```python
from build123d import *

# Parameters (mm, degrees)
PAD001_DEPTH     = 30
SKETCH003_W      = 15
SKETCH003_H      = 15
POCKET001_DEPTH  = 11.301
SKETCH004_R      = 2.5
PAD002_DEPTH     = 30
HOLE_D           = 4
HOLE_CSINK_D     = 8
HOLE_CSINK_ANGLE = 90
SKETCH006_R      = 2.65
POCKET002_DEPTH  = 30.001
FILLET001_R      = 1


with BuildPart() as part:
    # Sketch002 → Pad001 (new body)
    with BuildSketch(Plane.XY):
        with BuildLine():
            Line((120, 0), (138, 0))
            Line((138, 0), (138, 4))
            Line((138, 4), (125.403702, 4))
            ThreePointArc((125.403702, 4), (116.638453, 10.1912), (120, 0))
        make_face()
    extrude(amount=PAD001_DEPTH)

    # Sketch003 (on Face1 of Pad001) → Pocket001 (cut, through all)
    with BuildSketch(Plane.XZ):
        with Locations((118.3, 29.625)):
            Rectangle(SKETCH003_W, SKETCH003_H)
        with Locations((118.3, 0.375)):
            Rectangle(SKETCH003_W, SKETCH003_H)
    extrude(amount=-POCKET001_DEPTH, mode=Mode.SUBTRACT)

    # Sketch004 → Pad002 (join)
    with BuildSketch(Plane.XY):
        with Locations((120, 5.65)):
            Circle(SKETCH004_R)
    extrude(amount=PAD002_DEPTH)

    # Hole (through all)
    with Locations(Plane(origin=(0, 4, 0), x_dir=(-1, 0, 0), z_dir=(0, 1, 0))):
        with Locations((-131.9, 22.5), (-131.9, 7.5)):
            CounterSinkHole(HOLE_D / 2, HOLE_CSINK_D / 2, counter_sink_angle=HOLE_CSINK_ANGLE)

    # Sketch006 → Pocket002 (cut, through all)
    with BuildSketch(Plane.XY.offset(30)):
        with Locations((120, 5.65)):
            Circle(SKETCH006_R)
    extrude(amount=-POCKET002_DEPTH, mode=Mode.SUBTRACT)

    # Fillet001
    fillet001_edges = [part.edges().sort_by_distance(p)[0] for p in [
        (138, 4, 15),
        (131.9, 4, 0),
        (125.8, 4, 3.9375),
        (125.8, 4, 26.0625),
        (131.9, 4, 30),
    ]]
    fillet(fillet001_edges, radius=FILLET001_R)


solid = part.part
```
Here's how the part is built. I have some questions about the finished solid (model axes, mm). A direction names the side the tool comes from. Coordinates: 2 decimals unless noted, no trailing zeros. Order: outer loops, then holes, each group sorted by start corner. A loop starts at its lowest first (then second) coordinate and runs counter-clockwise, first axis right, second up. Notation, with made-up numbers: (21, 68) - (70, 68) arc R26 cw to (70, 83) - close; hole circle Ø8 at (-39, 36.5). An arc over 180 degrees is marked (long way). One line per question, with ' | ' between items. Start each with the question number.
1. If we mould it in two halves opening along X, with no side actions, what happens to faces 1 (the flat face through (132, 2, 0)), 2 (the cylindrical face through (137.699, 3.715, 15.21)), 3 (the cylindrical face through (122.528, 6.446, 15.1))? For each: released by +X, released by -X, zero draft, split by the parting line, or undercut.
2. If we section it at D-D (x = 118.75): Write out the boundary of the cut face in (y, z) (3 decimals), and give its area (3 significant figures).
3. I'm going to push flat-ended pins straight in: pin 1 Ø10 at (x, z) = (127.5, 17.5) entering from +Y; pin 2 Ø9.5 at (x, z) = (132.5, 18) entering from +Y; pin 3 Ø3 at (x, y) = (121, 2) entering from -Z (3 decimals). Where does each tip first touch, or does it pass through?
4. Please list where these lines run through material, in increasing order: line 1 along Z through (x, y) = (132, 1); line 2 along Z through (x, y) = (132.5, 3.5); line 3 along X through (y, z) = (1.05, 7.5). Write a range as [from, to].
5. If we section it at A-A (x = 131.9): Write out the boundary of the cut face in (y, z).
6. Which directions (+Z, -Z, +X, -X, +Y, -Y) give clear straight access to the entire face, cutting with the end or side of a thin tool? Please do faces 4 (the cylindrical face through (126.085, 3.699, 3.993)), 5 (the flat face through (125.8, 1, 26)), 6 (the cylindrical face through (126.101, 3.715, 26.118)).
7. If we section it at C-C (y = 6.5): Write out the boundary of the cut face in (x, z) (3 decimals), and give its area (3 significant figures).
8. If we section it at B-B (z = 22.5): Write out the boundary of the cut face in (x, y).
Model answer:
1) face 1: zero draft | face 2: released by +X | face 3: undercut
2) outline: (0.14, 7.875) - (3.313, 7.875) - (3.313, 22.125) - (0.14, 22.125) - close; (7.987, 7.875) - (11.16, 7.875) - (11.16, 22.125) - (7.987, 22.125) - close | area: 90.4 mm²
3) pin 1: stops at y = 10.72 | pin 2: stops at y = 4 | pin 3: stops at z = 7.875
4) line 1: z = [0, 5.5], [9.5, 20.5], [24.5, 30] | line 2: z = [0.13, 4.05], [10.95, 19.05], [25.95, 29.87] | line 3: x = [125.8, 129.9], [133.9, 138]
5) outline: (0, 0) - (3, 0) arc R1 ccw to (4, 1) - (4, 3.5) - (2, 5.5) - (0, 5.5) - close; (0, 9.5) - (2, 9.5) - (4, 11.5) - (4, 18.5) - (2, 20.5) - (0, 20.5) - close; (0, 24.5) - (2, 24.5) - (4, 26.5) - (4, 29) arc R1 ccw to (3, 30) - (0, 30) - close
6) face 4: -Z, -X, +Y | face 5: +Z, -X, +Y, -Y | face 6: +Z, -X, +Y
7) outline: (114.414, 7.875) - (117.49, 7.875) - (117.49, 22.125) - (114.414, 22.125) - close; (122.51, 7.875) - (125.586, 7.875) - (125.586, 22.125) - (122.51, 22.125) - close | area: 87.7 mm²
8) outline: (125.8, 0) - (129.9, 0) - (129.9, 2) - (127.9, 4) - (126.8, 4) arc R1 ccw to (125.8, 3) - close; (133.9, 0) - (138, 0) - (138, 3) arc R1 ccw to (137, 4) - (135.9, 4) - (133.9, 2) - close
